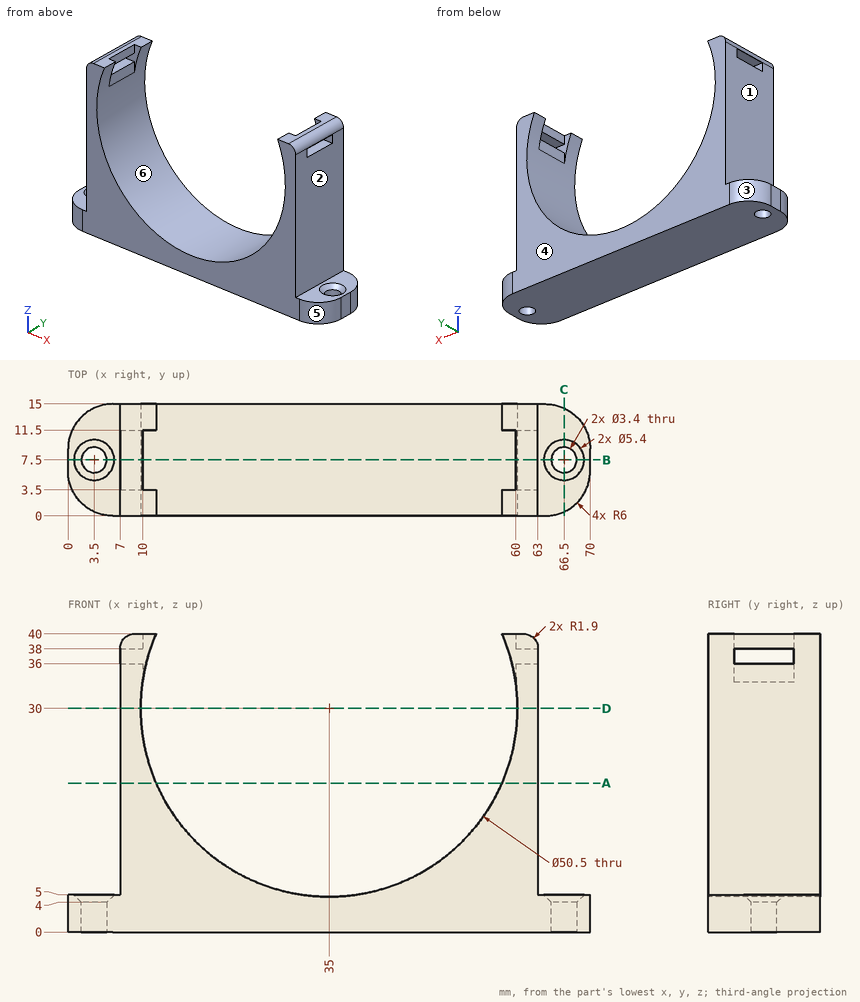
Geometry check sheet. Reference: drawing and pictorial views, mm from the part's lowest x, y, z. A direction names the side the tool comes from. Give positions to 0.01 mm unless a question says otherwise; leave off trailing zeros. Write each loop counter-clockwise with the first axis right and the second up, starting at its lowest first coordinate (ties: lowest second). Pieces come first, ordered by that corner, then holes. Notation, with made-up numbers: (33, 39) - (60, 39) arc R10 ccw to (60, 56) - close; hole circle Ø3 at (54, 81.5). An arc over 180 degrees is marked (long way). Put each result on its own line as item: value.
Q1. Section check A-A on z = 20. Record the cut outline in (x, y), and give its area (3 significant figures).
Result:
outline: (7, 0) - (11.81, 0) - (11.81, 15) - (7, 15) - close; (58.19, 0) - (63, 0) - (63, 15) - (58.19, 15) - close
area: 144 mm2
Q2. Set-up check for the marked faces 1, 2 and 3: record each of +Z, -Z, +X, -X, +Y, -Y from which the full face is reachable in a straight line by a thin tool's end or side.
Result:
face 1: +Z, -X, +Y, -Y
face 2: +Z, +X, +Y, -Y
face 3: +Z, -Z, -X, +Y
Q3. Section check B-B on y = 7.5. Count the separate pieces of the cut face and the enclosed holes in it, and give its area (3 significant figures).
Result:
separate pieces: 5
enclosed holes: 0
area: 758 mm2
Q4. Depth check by flat-ended pin: P1, Ø7.5, axis at x = 2, y = 7.5, coming from the +Z side; P2, Ø3, axis at y = 12, z = 35, coming from the +X side; P3, Ø1, axis at x = 29, y = 7, coming from the +Z side; P4, Ø2.5, axis at x = 3.5, y = 7.5, coming from the -Z side. Enter the tip coordinate at first touch or a pass-through.
Result:
P1: z = 5
P2: x = 63
P3: z = 5.6
P4: through
Q5. Section check C-C on x = 66.5. Record the cut outline in (y, z), and give its area (3 significant figures).
Result:
outline: (0.55, 0) - (5.8, 0) - (5.8, 4) - (4.8, 5) - (0.55, 5) - close; (9.2, 0) - (14.45, 0) - (14.45, 5) - (10.2, 5) - (9.2, 4) - close
area: 51.5 mm2
Q6. Scan lines: probe 1 along X at (y, z) = (11.25, 34.5); probe 2 along X at (y, z) = (1.25, 7); probe 3 along X at (y, z) = (5.75, 3.5). Record each from-to range of solid material in increasing order. Write a range as from..to.
Result:
probe 1: 7..10, 60..63
probe 2: 7..24.58, 45.42..63
probe 3: 0.01..69.99
Q7. Mould release check, pull along X, two halves, no side actions. Record for the marked faces 4, 5 and 6: released by +X, released by -X, zero draft, split by the parting line, or undercut.
Result:
face 4: zero draft
face 5: released by +X
face 6: undercut
Q8. Section check D-D on z = 30. Record the cut outline in (x, y).
Result:
outline: (7, 0) - (9.75, 0) - (9.75, 15) - (7, 15) - close; (60.25, 0) - (63, 0) - (63, 15) - (60.25, 15) - close
